from build123d import *

# Parameters (mm, degrees)
SKETCH_1_W          = 20
SKETCH_1_H          = 15
EXTRUDE_1_DEPTH     = 2.5
SKETCH_2_W          = 12.5
SKETCH_2_H          = 8.5
CUT_EXTRUDE_1_DEPTH = 6
CUT_EXTRUDE_2_REACH = 17
SKETCH_4_R          = 1.25


with BuildPart() as part:
    # 草圖1 → 填料-伸長1 (new body, symmetric)
    with BuildSketch(Plane.XY):
        Rectangle(SKETCH_1_W, SKETCH_1_H)
    extrude(amount=EXTRUDE_1_DEPTH, both=True)

    # 草圖2 → 除料-伸長1 (cut, through all)
    with BuildSketch(Plane.XY.offset(2.5)):
        Rectangle(SKETCH_2_W, SKETCH_2_H)
    extrude(amount=-CUT_EXTRUDE_1_DEPTH, mode=Mode.SUBTRACT)

    # 草圖4 → 除料-伸長2 (cut, up to next)
    with BuildSketch(Plane.XZ.offset(7.5), mode=Mode.PRIVATE) as cut_extrude_2_sk1:
        with Locations((-4, 0)):
            Circle(SKETCH_4_R)
    cut_extrude_2_tool1 = extrude(cut_extrude_2_sk1.sketch, amount=-CUT_EXTRUDE_2_REACH, mode=Mode.PRIVATE) & part.part
    add(cut_extrude_2_tool1.solids().sort_by_distance((-4, -7.5, 0))[0], mode=Mode.SUBTRACT)
    # 草圖4 → 除料-伸長2 (cut, up to next)
    with BuildSketch(Plane.XZ.offset(7.5), mode=Mode.PRIVATE) as cut_extrude_2_sk2:
        with Locations((4, 0)):
            Circle(SKETCH_4_R)
    cut_extrude_2_tool2 = extrude(cut_extrude_2_sk2.sketch, amount=-CUT_EXTRUDE_2_REACH, mode=Mode.PRIVATE) & part.part
    add(cut_extrude_2_tool2.solids().sort_by_distance((4, -7.5, 0))[0], mode=Mode.SUBTRACT)


solid = part.part
Read the model definition and answer for the solid it produces. Units are mm, in the model's axes. A direction names the side the tool comes from. Give positions to 0.01 mm unless a question says otherwise; leave off trailing zeros. Write each loop counter-clockwise with the first axis right and the second up, starting at its lowest first coordinate (ties: lowest second). Pieces come first, ordered by that corner, then holes. Notation, with made-up numbers: (-31, 87) - (-14, 87) arc R33 cw to (-14, 115) - close; hole circle Ø7 at (29.25, 49). An arc over 180 degrees is marked (long way). Return JSON: item names as keys, results as strings.
Q1. For a pull along X with two mould halves and no side action, classify faces 4 (the face through (0, -7.5, 0)), 5 (the face through (10, 0, 0)), 6 (the face through (5.19, -5.9, 0.38)) as released by +X, released by -X, zero draft, split by the parting line, or undercut.
Reply:
{"face 4": "zero draft", "face 5": "released by +X", "face 6": "undercut"}
Q2. A cutting plane is placed at D-D, the plane z = 1.85. Determine the outline of the cut face in (x, y), and give its area (3 significant figures).
Reply:
{"outline": "(-10, -7.5) - (10, -7.5) - (10, 7.5) - (-10, 7.5) - close; hole (-6.25, -4.25) - (6.25, -4.25) - (6.25, 4.25) - (-6.25, 4.25) - close", "area": "194 mm²"}
Q3. A cutting plane is placed at C-C, the plane x = 5. Determine the outline of the cut face in (y, z).
Reply:
{"outline": "(-7.5, -2.5) - (-4.25, -2.5) - (-4.25, -0.75) - (-7.5, -0.75) - close; (-7.5, 0.75) - (-4.25, 0.75) - (-4.25, 2.5) - (-7.5, 2.5) - close; (4.25, -2.5) - (7.5, -2.5) - (7.5, 2.5) - (4.25, 2.5) - close"}
Q4. For faces 1 (the face through (-5.25, -5.9, 0.05)), 2 (the face through (0, 7.5, 0)), 3 (the face through (6.25, 0, 0)), determine the directions among +Z, -Z, +X, -X, +Y, -Y from which every point of the face is accessible in a straight line to the end or side of a thin tool.
Reply:
{"face 1": "-Y", "face 2": "+Z, -Z, +X, -X, +Y", "face 3": "+Z, -Z"}
Q5. Consider line 1 along Z through (x, y) = (4, -5.25); line 2 along X through (y, z) = (-2, 1.8); line 3 along Y through (x, z) = (5, -1). Determine where each line is inside the solid, lowest interval first. Write a range as [from, to].
Reply:
{"line 1": "[-2.5, -1.25], [1.25, 2.5]", "line 2": "[-10, -6.25], [6.25, 10]", "line 3": "[-7.5, -4.25], [4.25, 7.5]"}
Q6. Given P1, Ø1, axis at x = 1.5, y = -4, coming from the +Z side; P2, Ø2, axis at x = -2, y = 2, coming from the +Z side; P3, Ø1.5, axis at x = 4, z = 0, coming from the -Y side, each flat-ended and moving along its own axis, determine where each tip first touches the part or whether it passes through.
Reply:
{"P1": "z = 2.5", "P2": "through", "P3": "y = 4.25"}
Q7. A cutting plane is placed at B-B, the plane z = 0. Determine the outline of the cut face in (x, y).
Reply:
{"outline": "(-10, -7.5) - (-5.25, -7.5) - (-5.25, -4.25) - (-6.25, -4.25) - (-6.25, 4.25) - (6.25, 4.25) - (6.25, -4.25) - (5.25, -4.25) - (5.25, -7.5) - (10, -7.5) - (10, 7.5) - (-10, 7.5) - close; (-2.75, -7.5) - (2.75, -7.5) - (2.75, -4.25) - (-2.75, -4.25) - close"}
Q8. A cutting plane is placed at A-A, the plane y = 0. Determine the outline of the cut face in (x, z), and give its area (3 significant figures).
Reply:
{"outline": "(-10, -2.5) - (-6.25, -2.5) - (-6.25, 2.5) - (-10, 2.5) - close; (6.25, -2.5) - (10, -2.5) - (10, 2.5) - (6.25, 2.5) - close", "area": "37.5 mm²"}
